Could you check a few things on this model? Use its own coordinates, in mm. Face numbers are marked on the shaded views. A direction names the side the tool comes from. Coordinates: 2 decimals unless noted, no trailing zeros. Order: outer loops, then holes, each group sorted by start corner. A loop starts at its lowest first (then second) coordinate and runs counter-clockwise, first axis right, second up. Notation, with made-up numbers: M -21,78.5 L 9,78.5 A25 cw 9,105.5 Z; hole C 24,-37.5 d11. An arc over 180 degrees is marked long. One line per question, with ' | ' between items. Start each with the question number.
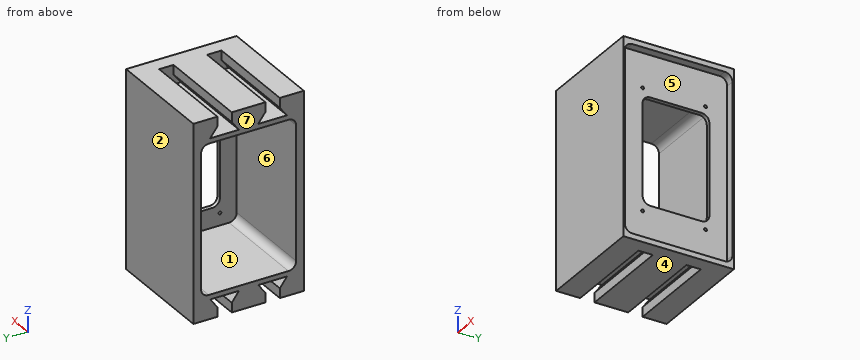
Autodesk Inventor part; units mm, degrees
ref_plane "YZ Plane" through (0, 0, 0) normal (1, 0, 0) x (0, 1, 0)
ref_plane "XZ Plane" through (0, 0, 0) normal (0, 1, 0) x (-1, 0, 0)
ref_plane "XY Plane" through (0, 0, 0) normal (0, 0, 1) x (1, 0, 0)
sketch "Sketch12" plane through (0, 0, 0) normal (0, 1, 0) x (-1, 0, 0)
  line L0 (0, 0) -> (0, -102.5) construction
  line L1 (0, 0) -> (0, 102.5) construction
  line L2 (0, 102.5) -> (125, 102.5) construction
  line L3 (125, 102.5) -> (125, -102.5) construction
  line L4 (125, -102.5) -> (0, -102.5) construction
  line L5 (0, -102.5) -> (0, 102.5) construction
  line L6 (0, 102.5) -> (45, 102.5) construction
  line L7 (45, 102.5) -> (45, -102.5) construction
  line L8 (45, -102.5) -> (0, -102.5) construction
  line L9 (0, -102.5) -> (0, 102.5) construction
  line L10 (125, 0) -> (125, -217.5) construction
  line L11 (125, 0) -> (125, 217.5) construction
  line L12 (125, 217.5) -> (72.0108, 217.5) construction
  line L13 (45, 217.5) -> (45, 102.5) construction
  line L14 (125, -217.5) -> (72.0108, -217.5) construction
  line L15 (45, -217.5) -> (45, -102.5) construction
  arc A0 (34.5307, 191.4729) -> (34.5307, -191.4729) centre (548.125, 0) ccw construction
  arc A1 (34.5307, -191.4729) -> (72.0108, -217.5) centre (72.0108, -177.5) ccw construction
  arc A2 (72.0108, 217.5) -> (34.5307, 191.4729) centre (72.0108, 177.5) ccw construction
  line L16 (125, -102.5) -> (125, 102.5)
  line L17 (125, 102.5) -> (9.6691, 102.5)
  line L18 (125, -102.5) -> (9.6691, -102.5)
  arc A3 (9.6691, 102.5) -> (9.6691, -102.5) centre (548.125, 0) ccw construction
  line L19 (9.6691, 102.5) -> (9.6691, -102.5)
  dimension "d698" = 102.5
  dimension "d699" = 102.5
  dimension "d700" = 125
  dimension "d701" = 45
  dimension "d702" = 217.5
  dimension "d703" = 217.5
  dimension "d704" = 40
extrude "Extrusion12" add sketch "Sketch12" along normal blind 115
sketch "Sketch84" plane through (-125, 0, -102.5) normal (-1, 0, 0) x (0, 0, 1)
  line L0 (33, 107) -> (172, 107)
  line L1 (180, 99) -> (180, 16)
  line L2 (172, 8) -> (33, 8)
  line L3 (25, 16) -> (25, 99)
  line L4 (205, 0) -> (205, 115)
  line L5 (0, 0) -> (0, 115)
  line L6 (0, 115) -> (205, 115)
  line L7 (0, 0) -> (205, 0)
  arc A0 (33, 107) -> (25, 99) centre (33, 99) ccw
  arc A1 (180, 99) -> (172, 107) centre (172, 99) ccw
  arc A2 (172, 8) -> (180, 16) centre (172, 16) ccw
  arc A3 (25, 16) -> (33, 8) centre (33, 16) ccw
  point P0 (102.5, 0)
  dimension "d705" = 25
  dimension "d706" = 25
  dimension "d707" = 8
  dimension "d708" = 8
  dimension "d709" = 8
extrude "Extrusion69" cut sketch "Sketch84" against normal blind 102 contours L0 A1 L1 A2 L2 A3 L3 A0
sketch "Sketch85" plane through (-125, 0, -102.5) normal (-1, 0, 0) x (0, 0, 1)
  line L0 (205, 0) -> (205, 97)
  line L1 (205, 25) -> (205, 40)
  line L2 (205, 32.5) -> (185, 32.5) construction
  line L3 (185, 32.5) -> (185, 47.5)
  line L4 (185, 32.5) -> (185, 17.5)
  line L5 (205, 40) -> (195, 40)
  line L6 (195, 40) -> (185, 47.5)
  line L7 (205, 25) -> (195, 25)
  line L8 (195, 25) -> (185, 17.5)
  line L9 (0, 0) -> (205, 0)
  line L10 (205, 75) -> (205, 90)
  line L11 (205, 82.5) -> (185, 82.5) construction
  line L12 (185, 82.5) -> (185, 97.5)
  line L13 (185, 82.5) -> (185, 67.5)
  line L14 (205, 75) -> (195, 75)
  line L15 (195, 75) -> (185, 67.5)
  line L16 (205, 90) -> (195, 90)
  line L17 (195, 90) -> (185, 97.5)
  line L18 (0, 115) -> (205, 115)
  line L19 (0, 0) -> (0, 115)
  line L20 (0, 25) -> (10, 25)
  line L21 (0, 25) -> (10, 25) construction
  line L22 (0, 25) -> (0, 40)
  line L23 (10, 40) -> (0, 40)
  line L24 (0, 32.5) -> (20, 32.5) construction
  line L25 (20, 32.5) -> (20, 47.5)
  line L26 (20, 47.5) -> (10, 40)
  line L27 (20, 32.5) -> (20, 17.5)
  line L28 (20, 17.5) -> (10, 25)
  line L29 (0, 90) -> (10, 90)
  line L30 (0, 90) -> (0, 75)
  line L31 (10, 75) -> (0, 75)
  line L32 (0, 82.5) -> (20, 82.5) construction
  line L33 (20, 82.5) -> (20, 97.5)
  line L34 (20, 97.5) -> (10, 90)
  line L35 (20, 82.5) -> (20, 67.5)
  line L36 (20, 67.5) -> (10, 75)
  point P0 (102.5, 0)
  dimension "d712" = 15
  dimension "d713" = 20
  dimension "d714" = 15
  dimension "d715" = 15
  dimension "d717" = 10
  dimension "d718" = 25
  dimension "d719" = 15
  dimension "d720" = 20
  dimension "d721" = 15
  dimension "d722" = 15
  dimension "d723" = 10
  dimension "d728" = 25
  dimension "d732" = 10
  dimension "d734" = 20
  dimension "d735" = 15
  dimension "d736" = 15
extrude "Extrusion70" cut sketch "Sketch85" against normal blind 100
sketch "Sketch86" plane through (-9.6691, 0, 102.5) normal (1, 0, 0) x (0, 0, -1)
  line L0 (0, 90) -> (0, 115) construction
  line L1 (0, 0) -> (205, 0) construction
  line L2 (0, 115) -> (205, 0) construction
  line L3 (0, 115) -> (205, 115) construction
  line L4 (205, 115) -> (0, 0) construction
  line L5 (191.5, 1.5) -> (13.5, 1.5)
  line L6 (5.5, 9.5) -> (5.5, 105.5)
  line L7 (13.5, 113.5) -> (191.5, 113.5)
  line L8 (199.5, 105.5) -> (199.5, 9.5)
  line L9 (199.5, 1.5) -> (5.5, 113.5) construction
  line L10 (5.5, 1.5) -> (199.5, 113.5) construction
  arc A0 (13.5, 113.5) -> (5.5, 105.5) centre (13.5, 105.5) ccw
  arc A1 (199.5, 105.5) -> (191.5, 113.5) centre (191.5, 105.5) ccw
  arc A2 (191.5, 1.5) -> (199.5, 9.5) centre (191.5, 9.5) ccw
  arc A3 (5.5, 9.5) -> (13.5, 1.5) centre (13.5, 9.5) ccw
  point P0 (102.5, 0)
  point P1 (102.5, 57.5)
  dimension "d738" = 194
  dimension "d739" = 112
  dimension "d740" = 8
extrude "Extrusion71" cut sketch "Sketch86" against normal blind 8.9
sketch "Sketch90" plane through (-18.5691, 0, 102.5) normal (1, 0, 0) x (0, 0, -1)
  circle A0 centre (41.2486, 90.9267) radius 1.5
  circle A1 centre (167.2486, 25.4267) radius 1.5
  circle A2 centre (41.2486, 25.4267) radius 1.5
  circle A3 centre (167.2486, 90.9267) radius 1.5
  line L0 (198.9986, 106.9003) -> (198.9986, 7.9003)
  line L1 (190.9986, 1.9267) -> (13.9986, 1.9267) construction
  line L2 (5.9986, 9.9267) -> (5.9986, 104.9267) construction
  line L3 (13.9986, 112.9267) -> (190.9986, 112.9267) construction
  line L4 (198.9986, 104.9267) -> (198.9986, 9.9267) construction
  arc A4 (13.9986, 112.9267) -> (5.9986, 104.9267) centre (13.9986, 104.9267) ccw
  arc A5 (198.9986, 104.9267) -> (190.9986, 112.9267) centre (190.9986, 104.9267) ccw
  arc A6 (190.9986, 1.9267) -> (198.9986, 9.9267) centre (190.9986, 9.9267) ccw
  arc A7 (5.9986, 9.9267) -> (13.9986, 1.9267) centre (13.9986, 9.9267) ccw
  line L5 (21.3986, 106.3267) -> (186.7486, 106.3267) construction
  line L6 (186.7486, 106.3267) -> (186.7486, 5.5767) construction
  line L7 (186.7486, 5.5767) -> (21.3986, 5.5767) construction
  line L8 (21.3986, 5.5767) -> (21.3986, 106.3267) construction
  line L9 (33.7486, 94.9267) -> (48.7486, 94.9267) construction
  line L10 (48.7486, 94.9267) -> (48.7486, 86.9267) construction
  line L11 (48.7486, 86.9267) -> (33.7486, 86.9267) construction
  line L12 (33.7486, 86.9267) -> (33.7486, 94.9267) construction
  line L13 (33.7486, 94.9267) -> (48.7486, 86.9267) construction
  line L14 (48.7486, 94.9267) -> (33.7486, 86.9267) construction
  line L15 (33.7486, 29.4267) -> (48.7486, 29.4267) construction
  line L16 (48.7486, 29.4267) -> (48.7486, 21.4267) construction
  line L17 (48.7486, 21.4267) -> (33.7486, 21.4267) construction
  line L18 (33.7486, 21.4267) -> (33.7486, 29.4267) construction
  line L19 (33.7486, 29.4267) -> (48.7486, 21.4267) construction
  line L20 (48.7486, 29.4267) -> (33.7486, 21.4267) construction
  line L21 (159.7486, 29.4267) -> (174.7486, 29.4267) construction
  line L22 (174.7486, 29.4267) -> (174.7486, 21.4267) construction
  line L23 (174.7486, 21.4267) -> (159.7486, 21.4267) construction
  line L24 (159.7486, 21.4267) -> (159.7486, 29.4267) construction
  line L25 (159.7486, 29.4267) -> (174.7486, 21.4267) construction
  line L26 (174.7486, 29.4267) -> (159.7486, 21.4267) construction
  line L27 (159.7486, 94.9267) -> (174.7486, 94.9267) construction
  line L28 (174.7486, 94.9267) -> (174.7486, 86.9267) construction
  line L29 (174.7486, 86.9267) -> (159.7486, 86.9267) construction
  line L30 (159.7486, 86.9267) -> (159.7486, 88.953) construction
  line L31 (159.7486, 94.9267) -> (174.7486, 86.9267) construction
  line L32 (174.7486, 94.9267) -> (159.7486, 86.9267) construction
  line L33 (159.7486, 94.9267) -> (159.7486, 84.9003) construction
  line L34 (56.7486, 94.9267) -> (151.7486, 94.9267)
  line L35 (159.7486, 86.9267) -> (159.7486, 33.4267)
  line L36 (151.7486, 25.4267) -> (56.7486, 25.4267)
  line L37 (48.7486, 33.4267) -> (48.7486, 86.9267)
  arc A8 (56.7486, 94.9267) -> (48.7486, 86.9267) centre (56.7486, 86.9267) ccw
  arc A9 (159.7486, 86.9267) -> (151.7486, 94.9267) centre (151.7486, 86.9267) ccw
  arc A10 (151.7486, 25.4267) -> (159.7486, 33.4267) centre (151.7486, 33.4267) ccw
  arc A11 (48.7486, 33.4267) -> (56.7486, 25.4267) centre (56.7486, 33.4267) ccw
  line L38 (0, 90) -> (0, 115) construction
  line L39 (205, 0) -> (205, 25) construction
  line L40 (0, 115) -> (205, 0) construction
  line L41 (205, 0) -> (205, 115) construction
  line L42 (0, 0) -> (0, 115) construction
  line L43 (0, 0) -> (205, 115) construction
  point P0 (102.5, 0)
  point P1 (5.9986, 112.9267)
  point P2 (5.9986, 1.9267)
  point P3 (198.9986, 112.9267)
  point P4 (159.7486, 25.4267)
  point P5 (102.4986, 57.5003)
  dimension "d840" = 3
  dimension "d841" = 3
  dimension "d842" = 3
  dimension "d843" = 3
  dimension "d844" = 193
  dimension "d845" = 111
  dimension "d846" = 8
  dimension "d847" = 8
  dimension "d848" = 165.35
  dimension "d849" = 100.75
  dimension "d850" = 3.65
  dimension "d851" = 15.4
  dimension "d852" = 15.4
  dimension "d853" = 19.85
  dimension "d854" = 19.85
  dimension "d855" = 15
  dimension "d856" = 8
  dimension "d857" = 15
  dimension "d858" = 15
  dimension "d859" = 8
  dimension "d860" = 19.5
  dimension "d861" = 19.85
  dimension "d862" = 19.5
  dimension "d863" = 19.85
  dimension "d864" = 12.25
  dimension "d865" = 0
  dimension "d866" = 8
  dimension "d868" = 15.4
  dimension "d869" = 6.6
  dimension "d870" = 12.25
extrude "Extrusion74" cut sketch "Sketch90" against normal blind 10
properties part number "center_fp13"
(1) We'd pull the mould along Y, two halves only. Please class the marked faces 1, 2, 3 and 4: +Y half, -Y half, draft (parallel to the pull), parting line (faces both ways), or undercut.
(2) Imagine slicing it at D-D, the plane y = 20. Write out the boundary of the cut face in (x, z).
(3) If I drill on line 1 along Y through (x, z) = (-98.5, 57); line 2 along Y through (x, z) = (-21.5, 5); line 3 along Z through (x, y) = (-31, 48), over which ranges is the centre line in solid material (lowest first)? Write a range as from..to.
(4) For P1, Ø15, axis at x = -93.5, y = 87.5, coming from the -Z side; P2, Ø2.5, axis at y = 90.93, z = -64.75, coming from the -X side; P3, Ø1, axis at x = -46.5, y = 33, coming from the -Z side; P4, Ø2, axis at x = -112, y = 80, coming from the +Z side, each with a flat end and sliding along its axis, tell me the tip position at first contact or that it passes through.
(5) Imagine slicing it at C-C, the plane y = 44.5. Write out the boundary of the cut face in (x, z), plus the area to 3 significant figures.
(6) On a 3-axis mill with a long thin cutter (end or side, diameter ignored), from which of +Z, -Z, +X, -X, +Y, -Y can I reach the whole of each face in a straight line? I mean the marked faces 5, 6 and 7. Say none if no direction works.
(7) Imagine slicing it at A-A, the plane z = 1. Write out the boundary of the cut face in (x, y), plus the area to 3 significant figures.
(8) Imagine slicing it at B-B, the plane y = 58. Write out the boundary of the cut face in (x, z), plus the area to 3 significant figures.
Answers:
1) face 1: undercut | face 2: +Y half | face 3: -Y half | face 4: draft
2) outline: M -125,-102.5 L -9.67,-102.5 L -9.67,-97 L -18.57,-97 L -18.57,97 L -9.67,97 L -9.67,102.5 L -125,102.5 L -125,85.83 L -25,85.83 L -25,82.5 L -125,82.5 L -125,77.5 L -23,77.5 L -23,-77.5 L -125,-77.5 L -125,-82.5 L -25,-82.5 L -25,-85.83 L -125,-85.83 Z
3) line 1: 0..8, 107..115 | line 2: 0..25.43, 94.93..115 | line 3: -102.5..-77.5, 77.5..102.5
4) P1: z = -102.5 | P2: through | P3: z = -82.5 | P4: z = 82.5
5) outline: M -125,-102.5 L -9.67,-102.5 L -9.67,-97 L -18.57,-97 L -18.57,-57.25 L -23,-57.25 L -23,-77.5 L -125,-77.5 L -125,-82.5 L -25,-82.5 L -25,-86.5 L -125,-86.5 Z; M -125,77.5 L -23,77.5 L -23,53.75 L -18.57,53.75 L -18.57,97 L -9.67,97 L -9.67,102.5 L -125,102.5 L -125,86.5 L -25,86.5 L -25,82.5 L -125,82.5 Z | area: 4,810 mm²
6) face 5: +X | face 6: -X | face 7: +Z, -Z, -X, +Y, -Y
7) outline: M -125,0 L -9.67,0 L -9.67,1.5 L -18.57,1.5 L -18.57,25.43 L -23,25.43 L -23,8 L -125,8 Z; M -125,107 L -23,107 L -23,94.93 L -18.57,94.93 L -18.57,113.5 L -9.67,113.5 L -9.67,115 L -125,115 Z | area: 1,860 mm²
8) outline: M -125,-102.5 L -9.67,-102.5 L -9.67,-97 L -18.57,-97 L -18.57,-57.25 L -23,-57.25 L -23,-77.5 L -125,-77.5 Z; M -125,77.5 L -23,77.5 L -23,53.75 L -18.57,53.75 L -18.57,97 L -9.67,97 L -9.67,102.5 L -125,102.5 Z | area: 5,610 mm²
